```python
from build123d import *

# Parameters (mm, degrees)
EXTRUSION1_DEPTH        = 0.81
ESQUISSE2_R             = 0.89
ENL_V_MAT_EXTRU_1_DEPTH = 0.81


with BuildPart() as part:
    # Esquisse1 → Extrusion1 (new body)
    with BuildSketch(Plane.XY):
        Polygon((-13.10407394, 11.361851996), (3.95592606, 11.361851996), (5.95592606, 9.361851996), (5.95592606, 2.471851996), (5.826054609, -1.342616085), (4.720113353, -1.342616085), (4.590241902, 2.471851996), (0.846236894, 2.471851996), (0.716236894, -1.338148004), (-0.293763106, -1.338148004), (-0.423763106, 2.471851996), (-6.18407394, 2.471851996), (-6.18407394, 5.011851996), (-13.10407394, 5.011851996), (-14.10407394, 6.011851996), (-14.10407394, 10.361851996), align=None)
    extrude(amount=EXTRUSION1_DEPTH)

    # Esquisse2 → Enlèv. mat.-Extru.1 (cut)
    with BuildSketch(Plane.XY.offset(0.81)):
        with Locations((-9.58407394, 8.186851996)):
            Circle(ESQUISSE2_R)
    extrude(amount=-ENL_V_MAT_EXTRU_1_DEPTH, mode=Mode.SUBTRACT)


solid = part.part
```
Can you work these out from the model? Positions are in its coordinate system, mm. A direction names the side the tool comes from. Give positions to 0.01 mm unless a question says otherwise; leave off trailing zeros. Order: outer loops, then holes, each group sorted by start corner. A loop starts at its lowest first (then second) coordinate and runs counter-clockwise, first axis right, second up. Notation, with made-up numbers: (16.5, 1.25) - (69.5, 1.25) arc R29 ccw to (69.5, 34.25) - close; hole circle Ø4 at (-5.75, 34). An arc over 180 degrees is marked (long way). Use a Markdown table: item, result. Add a question column.
Q1. On a 3-axis mill with a long thin cutter (end or side, diameter ignored), from which of +Z, -Z, +X, -X, +Y, -Y can I reach the whole of each face in a straight line? I mean faces 1 (the flat face through (2.7, 2.472, 0.4)), 2 (the flat face through (-14.104, 8.2, 0.4)), 3 (the flat face through (-9.6, 5.012, 0.4)). Say none if no direction works.
Q2. Please list where these lines run through material, in increasing order: line 1 along Y through (x, z) = (-0.5, 0.1); line 2 along Y through (x, z) = (-11.75, 0.35); line 3 along X through (y, z) = (3.5, 0.25).
Q3. If we section it at B-B on x = -9.75: Write out the boundary of the cut face in (y, z), plus the area to 3 significant figures.
Q4. If we section it at D-D on y = 4: Write out the boundary of the cut face in (x, z), plus the area to 3 significant figures.
Q5. If we mould it in two halves opening along X, with no side actions, what happens to faces 4 (the flat face through (4.94, 10.38, 0.4)), 5 (the cylindrical face through (-8.76, 7.85, 0.41)), 6 (the flat face through (-4.7, 11.362, 0.4))? For each: released by +X, released by -X, zero draft, split by the parting line, or undercut.
Q6. If we section it at C-C on z = 0.55: Write out the boundary of the cut face in (x, y), plus the area to 3 significant figures.
Q7. If we section it at A-A on y = -0.25: Write out the boundary of the cut face in (x, z).
Q8. I'm going to push a flat-ended pin straight in: pin 1 (6 mm diameter, centred on x = 3.5, y = 1.5, fed in from -Z). Where does the tip first touch, or does it pass through?
Answers follow:
| question | item | result |
|---|---|---|
| 1 | face 1 | +Z, -Z, -Y |
| 1 | face 2 | +Z, -Z, -X, +Y, -Y |
| 1 | face 3 | +Z, -Z, -X, -Y |
| 2 | line 1 | y = 2.47 to 11.36 |
| 2 | line 2 | y = 5.01 to 11.36 |
| 2 | line 3 | x = -6.18 to 5.96 |
| 3 | outline | (5.01, 0) - (7.31, 0) - (7.31, 0.81) - (5.01, 0.81) - close; (9.06, 0) - (11.36, 0) - (11.36, 0.81) - (9.06, 0.81) - close |
| 3 | area | 3.73 mm^2 |
| 4 | outline | (-6.18, 0) - (5.96, 0) - (5.96, 0.81) - (-6.18, 0.81) - close |
| 4 | area | 9.83 mm^2 |
| 5 | face 4 | released by +X |
| 5 | face 5 | undercut |
| 5 | face 6 | zero draft |
| 6 | outline | (-14.1, 6.01) - (-13.1, 5.01) - (-6.18, 5.01) - (-6.18, 2.47) - (-0.42, 2.47) - (-0.29, -1.34) - (0.72, -1.34) - (0.85, 2.47) - (4.59, 2.47) - (4.72, -1.34) - (5.83, -1.34) - (5.96, 2.47) - (5.96, 9.36) - (3.96, 11.36) - (-13.1, 11.36) - (-14.1, 10.36) - close; hole circle Ø1.78 at (-9.58, 8.19) |
| 6 | area | 162 mm^2 |
| 7 | outline | (-0.33, 0) - (0.75, 0) - (0.75, 0.81) - (-0.33, 0.81) - close; (4.68, 0) - (5.86, 0) - (5.86, 0.81) - (4.68, 0.81) - close |
| 8 | pin 1 | stops at z = 0 |
